```python
from build123d import *

# Parameters (mm, degrees)
SKETCH1_W           = 121.92
SKETCH1_H           = 173.482
BOSS_EXTRUDE1_DEPTH = 6.35
SKETCH2_R           = 3
BOSS_EXTRUDE2_DEPTH = 44.45
FILLET1_R           = 6.35
FILLET2_R           = 3.81


with BuildPart() as part:
    # Sketch1 → Boss-Extrude1 (new body)
    with BuildSketch(Plane(origin=(0, 0, 0), x_dir=(1, 0, 0), z_dir=(0, 1, 0))):
        with Locations((54.61, 80.391)):
            Rectangle(SKETCH1_W, SKETCH1_H)
    extrude(amount=BOSS_EXTRUDE1_DEPTH)

    # Sketch2 → Boss-Extrude2 (add)
    with BuildSketch(Plane(origin=(0, 6.35, 0), x_dir=(1, 0, 0), z_dir=(0, 1, 0))):
        with Locations((104.14, 5.08)):
            Circle(SKETCH2_R)
        with Locations((104.14, 123.19)):
            Circle(SKETCH2_R)
        with Locations((5.08, 123.19)):
            Circle(SKETCH2_R)
        with Locations((5.08, 5.08)):
            Circle(SKETCH2_R)
    extrude(amount=BOSS_EXTRUDE2_DEPTH)

    # Fillet1
    fillet1_edges = [part.edges().sort_by_distance(p)[0] for p in [
        (-6.35, 3.175, -167.132),
        (115.57, 3.175, -167.132),
        (115.57, 3.175, 6.35),
        (-6.35, 3.175, 6.35),
    ]]
    fillet(fillet1_edges, radius=FILLET1_R)

    # Fillet2
    fillet2_edges = [part.edges().sort_by_distance(p)[0] for p in [
        (101.14, 6.35, -5.08),
        (101.14, 6.35, -123.19),
        (2.08, 6.35, -123.19),
        (2.08, 6.35, -5.08),
    ]]
    fillet(fillet2_edges, radius=FILLET2_R)

    # Sketch3 → Revolve1 (revolve)
    with BuildSketch(Plane.XY.offset(-5.08)):
        Polygon((3.880000114, 50.8), (5.08, 50.8), (5.08, 54.499999886), (3.880000114, 53.3), align=None)
    revolve1 = revolve(axis=Axis((5.08, 50.8, -5.08), (0, -1, 0)))

    # Mirror1: Revolve1 across plane
    add(revolve1.mirror(Plane.XY.offset(-64.135)))

    # Mirror2: Revolve1 across plane
    add(revolve1.mirror(Plane.ZY.offset(-54.61)))

    # Mirror2 copy 1 sketch → Mirror2 copy 1 (revolve)
    with BuildSketch(Plane(origin=(109.22, 0, -123.19), x_dir=(-1, 0, 0), z_dir=(0, 0, -1))):
        Polygon((3.880000114, 50.8), (5.08, 50.8), (5.08, 54.499999886), (3.880000114, 53.3), align=None)
    revolve(axis=Axis((104.14, 50.8, -123.19), (0, -1, 0)))


solid = part.part
```
Part model, mm, in its own coordinate system. A direction names the side the tool comes from. Round coordinates to 2 decimals unless told otherwise and drop trailing zeros. Loops run counter-clockwise (first coordinate to the right, second up) from the corner with the lowest first, then second, coordinate; pieces in that order, holes last.
Item 1: Cut at A-A, the plane y = 29.5. Give the cut face in (x, z), then the cut area to 3 significant figures.
Item 2: Drop flat-ended pins along their axis: P1, Ø12, axis at x = 52.5, z = -26, coming from the +Y side; P2, Ø1.8, axis at x = 6, z = -122.5, coming from the +Y side; P3, Ø2, axis at y = 43, z = -119.5, coming from the -X side; P4, Ø1, axis at x = 42.5, y = 7.5, coming from the +Z side. Give the stop position or say it passes through.
Item 3: Drill centre lines: line 1 (Y direction, x = 88, z = -93); line 2 (Z direction, x = 3.5, y = 22.5); line 3 (X direction, y = 34, z = -125.5). Where is each one in solid material? Low to high.
Item 4: 3-axis set-ups, long thin cutter, end or side, ignore diameter. For faces 4 (the face through (105.524, 30.196, -120.528)), 5 (the face through (113.7, 3.2, 4.5)): which of +Z, -Z, +X, -X, +Y, -Y reach the whole face in a straight line?
Item 5: Cut at B-B, the plane x = 28. Give the cut face in (y, z).
Item 6: Mould opens along X. For faces 1 (the face through (115.57, 3, -79)), 2 (the face through (54, 0, -82)), 3 (the face through (105, 50.8, -4)) say: +X half, -X half, draft (parallel to the pull), parting line (faces both ways), or undercut.
Item 7: Cut at C-C, the plane z = -81.5. Give the cut face in (x, y).
A:
1. outline: circle Ø6 at (5.08, -123.19); circle Ø6 at (5.08, -5.08); circle Ø6 at (104.14, -123.19); circle Ø6 at (104.14, -5.08)
1. area: 113 mm2
2. P1: stops at y = 6.35
2. P2: stops at y = 54.25
2. P3: stops at x = 3.75
2. P4: passes through
3. line 1: y = 0 to 6.35
3. line 2: z = -125.74 to -120.64, -7.63 to -2.53
3. line 3: x = 3.17 to 6.99, 102.23 to 106.05
4. face 4: +Y
4. face 5: +Z, +X, +Y, -Y
5. outline: (0, -167.13) - (6.35, -167.13) - (6.35, 6.35) - (0, 6.35) - close
6. face 1: +X half
6. face 2: draft
6. face 3: undercut
7. outline: (-6.35, 0) - (115.57, 0) - (115.57, 6.35) - (-6.35, 6.35) - close
